The listing builds one solid part. Answer for the finished solid, in the listing's coordinates (mm). A direction names the side the tool comes from. Give positions to 0.01 mm unless a question says otherwise; leave off trailing zeros. Write each loop counter-clockwise with the first axis right and the second up, starting at its lowest first coordinate (ties: lowest second). Pieces come first, ordered by that corner, then holes. Notation, with made-up numbers: (-37.5, 47.25) - (-6.5, 47.25) arc R33 cw to (-6.5, 86.25) - close; hole circle Ø6 at (12, 52.5). An arc over 180 degrees is marked (long way). Answer as CSV lines item,"result". Start each with the question number.
(1) Find section D-D (x = -110). Write down the section's boundary in (y, z), then the cut area to 3 significant figures.
(2) Straight lines are drawn through the part: probe 1 along Y at (x, z) = (75, 62.85); probe 2 along X at (y, z) = (-53, 62.55); probe 3 along Y at (x, z) = (-5.5, 59.5). For each, find the intervals that lie inside material, in ascending order.
(3) For a pull along Y with two mould halves and no side action, classify faces 3 (the face through (-125, -1, 32)), 4 (the face through (121, -1, 30)), 5 (the face through (-2, 75, 32)) as pulls with the +Y half, pulls with the -Y half, needs draft (parallel to the pull), parting line crosses it, or undercut.
(4) Find section C-C (z = 10). Write down the section's boundary in (x, y).
(5) Find section B-B (y = 13). Write down the section's boundary in (x, z).
(6) Find section A-A (x = -54.5). Write down the section's boundary in (y, z), then the cut area to 3 significant figures.
(7) For faces 1 (the face through (-121, -1, 30)), 2 (the face through (125, -1, 32)), determine the directions among +Z, -Z, +X, -X, +Y, -Y from which every point of the face is accessible in a straight line to the end or side of a thin tool.
from build123d import *

# Parameters (mm, degrees)
F0_W     = 250
F0_H     = 150
F1_DEPTH = 64
F2_T     = -4
F3_W     = 140
F3_H     = 123
F3_R     = 2
F4_DEPTH = 64.001


with BuildPart() as f1:
    # F0 (on Top) → F1 (new body)
    with BuildSketch(Plane.XY):
        Rectangle(F0_W, F0_H)
    extrude(amount=F1_DEPTH)

    # F2
    f2_openings = [f1.faces().sort_by_distance(p)[0] for p in [
        (0, 0, 0),
    ]]
    offset(amount=F2_T, openings=f2_openings)

    # F3 (on Top) → F4 (cut, through all)
    with BuildSketch(Plane.XY):
        Rectangle(F3_W, F3_H)
        with Locations((-75, -53)):
            Circle(F3_R)
        with Locations((75, -53)):
            Circle(F3_R)
        with Locations((-75, 53)):
            Circle(F3_R)
        with Locations((75, 53)):
            Circle(F3_R)
    extrude(amount=F4_DEPTH, mode=Mode.SUBTRACT)


solid = f1.part
Result set:
1,outline,"(-75, 0) - (-71, 0) - (-71, 60) - (71, 60) - (71, 0) - (75, 0) - (75, 64) - (-75, 64) - close"
1,area,"1,080 mm^2"
2,probe 1,"-75 to -55, -51 to 51, 55 to 75"
2,probe 2,"-125 to -77, -73 to -70, 70 to 73, 77 to 125"
2,probe 3,"-75 to -71, 71 to 75"
3,face 3,"needs draft"
3,face 4,"undercut"
3,face 5,"pulls with the +Y half"
4,outline,"(-125, -75) - (125, -75) - (125, 75) - (-125, 75) - close; hole (-121, -71) - (121, -71) - (121, 71) - (-121, 71) - close"
5,outline,"(-125, 0) - (-121, 0) - (-121, 60) - (-70, 60) - (-70, 64) - (-125, 64) - close; (70, 60) - (121, 60) - (121, 0) - (125, 0) - (125, 64) - (70, 64) - close"
6,outline,"(-75, 0) - (-71, 0) - (-71, 60) - (-61.5, 60) - (-61.5, 64) - (-75, 64) - close; (61.5, 60) - (71, 60) - (71, 0) - (75, 0) - (75, 64) - (61.5, 64) - close"
6,area,"588 mm^2"
7,face 1,"-Z"
7,face 2,"+Z, -Z, +X, +Y, -Y"
